Geometry check sheet. Reference: the model listing, model coordinates, mm. A direction names the side the tool comes from. Coordinates: 2 decimals unless noted, no trailing zeros. Write each loop counter-clockwise with the first axis right and the second up, starting at its lowest first coordinate (ties: lowest second). Pieces come first, ordered by that corner, then holes. Notation, with made-up numbers: M 28,22.25 L 59,22.25 A12 cw 59,32.25 Z; hole C 1,5 d11. An arc over 180 degrees is marked long. Put each result on its own line as item: value. Start each with the question number.
1) Set-up check for faces 1 (the flat face through (9, 0, 12.7)), 2 (the flat face through (9, 0, -11.112)): record each of +Z, -Z, +X, -X, +Y, -Y from which the full face is reachable in a straight line by a thin tool's end or side.
2) Mould release check, pull along Y, two halves, no side actions. Record for faces 3 (the flat face through (9, 12.7, 0)), 4 (the flat face through (-609.6, 0.1, 11.3)), 5 (the flat face through (9, -11.112, 0)): released by +Y, released by -Y, zero draft, split by the parting line, or undercut.
3) Cross-section at B-B on y = 0. Count the separate pieces of the cut face and the enclosed holes in it, plus the area to 3 significant figures.
4) Scan lines: line 1 along Y through (x, z) = (-45, -7.5); line 2 along Z through (x, y) = (0, 11.75). Record each from-to range of solid material in increasing order.
5) Cross-section at A-A on x = 142. Record the cut outline in (y, z), plus the area to 3 significant figures.
from build123d import *

# Parameters (mm, degrees)
SKETCH1_W                  = 25.4
SKETCH1_H                  = 25.4
SKETCH1_W_2                = 22.225
SKETCH1_H_2                = 22.225
EXTRUDE_THIN1_DEPTH        = 609.6
F_1_2_0_5_DIAMETER_HOLE1_D = 12.7
F_1_4_CLEARANCE_HOLE1_D    = 6.7564


with BuildPart() as part:
    # Sketch1 → Extrude-Thin1 (new, symmetric)
    with BuildSketch(Plane(origin=(0, 0, 0), x_dir=(0, 0, -1), z_dir=(1, 0, 0))):
        Rectangle(SKETCH1_W, SKETCH1_H)
        Rectangle(SKETCH1_W_2, SKETCH1_H_2, mode=Mode.SUBTRACT)
    extrude(amount=EXTRUDE_THIN1_DEPTH, both=True)

    # 1/2 (0.5) Diameter Hole1 (through all)
    with Locations(Plane.XY.offset(12.7)):
        with Locations((-593.725, 0), (593.725, 0), (-92.075, 0)):
            Hole(F_1_2_0_5_DIAMETER_HOLE1_D / 2)

    # 1/4 Clearance Hole1 (through all)
    with Locations(Plane(origin=(0, 12.7, 0), x_dir=(1, 0, 0), z_dir=(0, 1, 0))):
        with Locations((-508, 0), (0, 0), (508, 0)):
            Hole(F_1_4_CLEARANCE_HOLE1_D / 2)


solid = part.part
Answer key:
1. face 1: +Z, +X, -X, +Y, -Y
1. face 2: +X, -X
2. face 3: released by +Y
2. face 4: zero draft
2. face 5: undercut
3. separate pieces: 8
3. enclosed holes: 0
3. area: 3,750 mm²
4. line 1: y = -12.7 to -11.11, 11.11 to 12.7
4. line 2: z = -12.7 to -3.38, 3.38 to 12.7
5. outline: M -12.7,-12.7 L 12.7,-12.7 L 12.7,12.7 L -12.7,12.7 Z; hole M -11.11,-11.11 L 11.11,-11.11 L 11.11,11.11 L -11.11,11.11 Z
5. area: 151 mm²
